```python
from build123d import *

# Parameters (mm, degrees)
BOSS_EXTRUDE1_DEPTH                       = 3.175
SKETCH2_R                                 = 5.0419
CUT_EXTRUDE1_DEPTH                        = 4.175
F_4_CLEARANCE_HOLE1_D                     = 3.4544
F_10_CLEARANCE_HOLE1_D                    = 5.6134
F_4_CLEARANCE_HOLE2_D                     = 3.4544
F_27_64_0_42188_DIAMETER_HOLE1_D          = 10.715752
F_3_32_0_09375_DIAMETER_HOLE1_D           = 2.38125
F_10_CLEARANCE_HOLE2_D                    = 5.6134
SKETCH15_W                                = 148.719955274
SKETCH15_H                                = 114.3
BOSS_EXTRUDE2_DEPTH                       = 3.175
CHAMFER1_SIZE                             = 2.54
F_10_CLEARANCE_HOLE3_D                    = 5.6134
CSK_FOR_8_FLAT_HEAD_MACHINE_SCREW_2_COUNT = 2
CSK_FOR_8_FLAT_HEAD_MACHINE_SCREW_2_PITCH = 30.13075


with BuildPart() as part:
    # Sketch1 → Boss-Extrude1 (new body)
    with BuildSketch(Plane.XY):
        with BuildLine():
            Line((-37.014245685, -65.193042462), (-37.014245685, -242.993042462))
            Line((-37.014245685, -242.993042462), (111.705709589, -242.993042462))
            Line((111.705709589, -242.993042462), (111.705709589, -78.837199032))
            Line((111.705709589, -78.837199032), (100.315919098, -73.219132409))
            Line((100.315919098, -73.219132409), (98.04889923, -77.407452736))
            ThreePointArc((98.04889923, -77.407452736), (95.944511883, -76.292837527), (93.820355363, -75.216374688))
            Line((93.820355363, -75.216374688), (91.991959695, -69.073183497))
            Line((91.991959695, -69.073183497), (87.625459733, -67.171845985))
            Line((87.625459733, -67.171845985), (85.800454124, -71.570795948))
            ThreePointArc((85.800454124, -71.570795948), (33.712742218, -61.505341345), (-18.130011823, -72.76464689))
            Line((-18.130011823, -72.76464689), (-20.055584156, -68.408779876))
            Line((-20.055584156, -68.408779876), (-21.49685031, -65.148469374))
            Line((-21.49685031, -65.148469374), (-28.430836618, -65.168386968))
            Line((-28.430836618, -65.168386968), (-37.014245685, -65.193042462))
        make_face()
    extrude(amount=-BOSS_EXTRUDE1_DEPTH)

    # Sketch2 → Cut-Extrude1 (cut, through all)
    with BuildSketch(Plane.XY):
        with Locations((35.268404938, -193.371995598)):
            Circle(SKETCH2_R)
    extrude(amount=-CUT_EXTRUDE1_DEPTH, mode=Mode.SUBTRACT)

    # #4 Clearance Hole1 (through all)
    with Locations(Plane.XY):
        with Locations((41.939844363, -71.488811907), (9.789450293, -73.011273216), (90.488583573, -124.967078721), (53.658735514, -125.072870965), (25.338848707, -124.341705755), (-9.634401538, -135.888162669), (55.145248163, -67.700310852), (3.101953943, -70.270684884)):
            Hole(F_4_CLEARANCE_HOLE1_D / 2)

    # #10 Clearance Hole1 (through all)
    with Locations(Plane.XY):
        with Locations((-29.394245685, -79.071995598), (104.085709589, -87.326995598), (35.695953558, -148.921995598), (26.485754315, -79.071995598)):
            Hole(F_10_CLEARANCE_HOLE1_D / 2)

    # #4 Clearance Hole2 (through all)
    with Locations(Plane.XY):
        with Locations((-8.073739309, -116.319383279), (-22.812224861, -96.782058908), (-10.478566815, -201.738004366), (-4.603970045, -177.980497914)):
            Hole(F_4_CLEARANCE_HOLE2_D / 2)

    # 27/64 (0.42188) Diameter Hole1 (through all)
    with Locations(Plane.XY):
        with Locations((81.551198953, -216.670082089)):
            Hole(F_27_64_0_42188_DIAMETER_HOLE1_D / 2)

    # 3/32 (0.09375) Diameter Hole1 (through all)
    with Locations(Plane.XY):
        with Locations((81.551198953, -224.036082089)):
            Hole(F_3_32_0_09375_DIAMETER_HOLE1_D / 2)

    # #10 Clearance Hole2 (through all)
    with Locations(Plane.XY):
        with Locations((-29.076745685, -192.193042462), (103.768209589, -211.243042462)):
            Hole(F_10_CLEARANCE_HOLE2_D / 2)

    # Sketch15 → Boss-Extrude2 (add, through all)
    with BuildSketch(Plane.XY):
        with Locations((37.345731952, -300.143042462)):
            Rectangle(SKETCH15_W, SKETCH15_H)
    extrude(amount=-BOSS_EXTRUDE2_DEPTH)

    # Chamfer1
    chamfer1_edges = [part.edges().sort_by_distance(p)[0] for p in [
        (-37.014245685, -357.293042462, -1.5875),
        (111.705709589, -357.293042462, -1.5875),
    ]]
    chamfer(chamfer1_edges, length=CHAMFER1_SIZE)

    # #10 Clearance Hole3 (through all)
    with Locations(Plane.XY):
        with Locations((95.830709589, -341.418042462), (37.345731952, -341.418042462), (-21.139245685, -341.418042462), (95.830709589, -290.618042462), (-21.139245685, -290.618042462)):
            Hole(F_10_CLEARANCE_HOLE3_D / 2)

    # Sketch19 → CSK for #8 Flat Head Machine Screw (100)2 (revolve, cut)
    with BuildSketch(Plane(origin=(20.203029938, -193.371995598, 0), x_dir=(0, -1, 0), z_dir=(1, 0, 0))):
        Polygon((0, 0), (0, 3.175), (2.45745, 3.175), (2.45745, 1.475934296), (4.2164, 0), align=None)
    csk_for_8_flat_head_machine_screw_100 = revolve(axis=Axis((20.203029938, -193.371995598, 6.35), (0, 0, -1)), mode=Mode.SUBTRACT)

    # CSK for _8 Flat Head Machine Screw _ 2: CSK for #8 Flat Head Machine Screw (100)2 ×2
    with Locations(*[(i * CSK_FOR_8_FLAT_HEAD_MACHINE_SCREW_2_PITCH, 0, 0) for i in range(1, CSK_FOR_8_FLAT_HEAD_MACHINE_SCREW_2_COUNT)]):
        add(csk_for_8_flat_head_machine_screw_100, mode=Mode.SUBTRACT)


solid = part.part
```
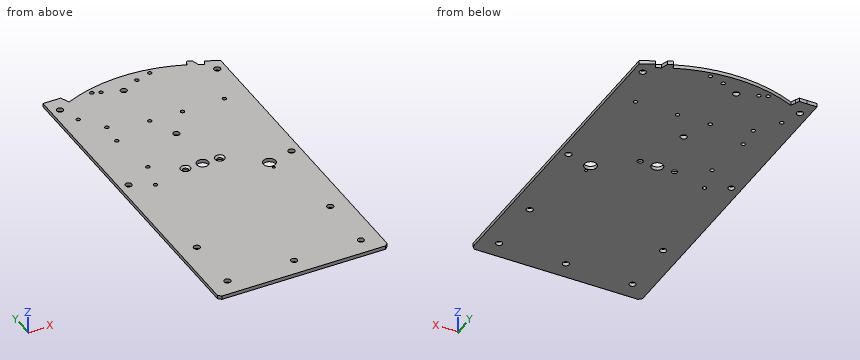
Input: part model. Units: mm. Frame: model coordinates. Coordinates: 2 decimals unless noted, no trailing zeros. Loops run counter-clockwise (first coordinate to the right, second up) from the corner with the lowest first, then second, coordinate; pieces in that order, holes last. Notation, with made-up numbers: M 29.25,87 L 79.25,87 A18 ccw 79.25,108 Z; hole C 27.5,28 d5. An arc over 180 degrees is marked long. One line per item, written item: value.
(1) Line query: line 1 along Y through (x, z) = (37, -1.4); line 2 along Y through (x, z) = (-10, -2.8); line 3 along Y through (x, z) = (80, -1.4). Output: solid intervals per line, ascending. Write a range as from..to.
Filled in:
line 1: -357.29..-344.2, -338.63..-198.11, -188.64..-151.41, -146.44..-61.51
line 2: -357.29..-203.4, -200.08..-137.58, -134.2..-69.49
line 3: -357.29..-221.8, -211.54..-69.32
(2) Section B-B (x = 73.5). Output: boundary loops of the cut face in (y, z) (3 decimals), and give its area (3 significant figures).
Filled in:
outline: M -357.293,-3.175 L -67.168,-3.175 L -67.168,0 L -357.293,0 Z
area: 921 mm^2
(3) Section A-A (z = -2.4). Give the number of separate pieces and of enclosed holes in the cut face, and give its area (3 significant figures).
Filled in:
separate pieces: 1
enclosed holes: 28
area: 42,600 mm^2
(4) Pin query (flat end, axial travel): pin 1 (3 mm diameter, centred on x = 90.49, y = -124.97, fed in from +Z). Return the tip coordinate at first contact, or that it passes through.
Filled in:
pin 1: through
